Source: CAD feature listing. Evaluate the final solid. Frame: model axes, mm. A direction names the side the tool comes from. Give positions to 0.01 mm unless a question says otherwise; leave off trailing zeros. Order: outer loops, then holes, each group sorted by start corner. A loop starts at its lowest first (then second) coordinate and runs counter-clockwise, first axis right, second up. Notation, with made-up numbers: M 45,38 L 73,38 A20 cw 73,74 Z; hole C -7.5,-11 d5. An arc over 180 degrees is marked long. Return JSON: item names as keys, results as strings.
from build123d import *

# Parameters (mm, degrees)
SKETCH1_W           = 440
SKETCH1_H           = 170
BOSS_EXTRUDE1_DEPTH = 25
SKETCH2_R           = 9.5
CUT_EXTRUDE1_DEPTH  = 15
SKETCH4_R           = 6
CUT_EXTRUDE3_DEPTH  = 237.326045962
SKETCH3_R           = 9.5
CUT_EXTRUDE2_DEPTH  = 15
SKETCH5_R           = 6
CUT_EXTRUDE4_DEPTH  = 237.326045962


with BuildPart() as part:
    # Sketch1 → Boss-Extrude1 (new body)
    with BuildSketch(Plane.XY):
        Rectangle(SKETCH1_W, SKETCH1_H)
    extrude(amount=BOSS_EXTRUDE1_DEPTH)

    # Sketch2 → Cut-Extrude1 (cut)
    with BuildSketch(Plane.XY.offset(25)):
        with Locations((170, 65)):
            Circle(SKETCH2_R)
        with Locations((45, 65)):
            Circle(SKETCH2_R)
        with Locations((-80, 65)):
            Circle(SKETCH2_R)
        with Locations((-205, 65)):
            Circle(SKETCH2_R)
        with Locations((45, -60)):
            Circle(SKETCH2_R)
        with Locations((-80, -60)):
            Circle(SKETCH2_R)
        with Locations((-205, -60)):
            Circle(SKETCH2_R)
        with Locations((170, -60)):
            Circle(SKETCH2_R)
    extrude(amount=-CUT_EXTRUDE1_DEPTH, mode=Mode.SUBTRACT)

    # Sketch4 → Cut-Extrude3 (cut, through all)
    with BuildSketch(Plane.XY.offset(10)):
        with Locations((170, 65)):
            Circle(SKETCH4_R)
        with Locations((45, 65)):
            Circle(SKETCH4_R)
        with Locations((-80, 65)):
            Circle(SKETCH4_R)
        with Locations((-205, 65)):
            Circle(SKETCH4_R)
        with Locations((45, -60)):
            Circle(SKETCH4_R)
        with Locations((-80, -60)):
            Circle(SKETCH4_R)
        with Locations((-205, -60)):
            Circle(SKETCH4_R)
        with Locations((170, -60)):
            Circle(SKETCH4_R)
    extrude(amount=-CUT_EXTRUDE3_DEPTH, mode=Mode.SUBTRACT)

    # Sketch3 → Cut-Extrude2 (cut)
    with BuildSketch(Plane(origin=(0, 0, 0), x_dir=(-1, 0, 0), z_dir=(0, 0, -1))):
        with Locations((-107.5, -60)):
            Circle(SKETCH3_R)
        with Locations((17.5, -60)):
            Circle(SKETCH3_R)
        with Locations((142.5, -60)):
            Circle(SKETCH3_R)
        with Locations((17.5, 65)):
            Circle(SKETCH3_R)
        with Locations((142.5, 65)):
            Circle(SKETCH3_R)
        with Locations((-107.5, 65)):
            Circle(SKETCH3_R)
    extrude(amount=-CUT_EXTRUDE2_DEPTH, mode=Mode.SUBTRACT)

    # Sketch5 → Cut-Extrude4 (cut, through all)
    with BuildSketch(Plane(origin=(0, 0, 15), x_dir=(-1, 0, 0), z_dir=(0, 0, -1))):
        with Locations((-107.5, -60)):
            Circle(SKETCH5_R)
        with Locations((17.5, -60)):
            Circle(SKETCH5_R)
        with Locations((142.5, -60)):
            Circle(SKETCH5_R)
        with Locations((17.5, 65)):
            Circle(SKETCH5_R)
        with Locations((142.5, 65)):
            Circle(SKETCH5_R)
        with Locations((-107.5, 65)):
            Circle(SKETCH5_R)
    extrude(amount=-CUT_EXTRUDE4_DEPTH, mode=Mode.SUBTRACT)


solid = part.part
1. Section query A-A (x = -17.5). Return loops of the section in (y, z).
Evaluation:
{"outline": "M -85,0 L -69.5,0 L -69.5,15 L -66,15 L -66,25 L -85,25 Z; M -54,15 L -50.5,15 L -50.5,0 L 55.5,0 L 55.5,15 L 59,15 L 59,25 L -54,25 Z; M 71,15 L 74.5,15 L 74.5,0 L 85,0 L 85,25 L 71,25 Z"}
2. Ray query, probe 1 along Y at (x, z) = (170, 14); probe 2 along Y at (x, z) = (45, 2). Return the intervals inside material, ascending.
Evaluation:
{"probe 1": "y = -85 to -69.5, -50.5 to 55.5, 74.5 to 85", "probe 2": "y = -85 to -66, -54 to 59, 71 to 85"}
3. First-contact query: pin 1 (15 mm diameter, centred on x = -142.5, y = 65, fed in from -Z); pin 2 (15.5 mm diameter, centred on x = -80, y = -60, fed in from +Z). Flat tips, straight axial feed; report the tip coordinate or a pass-through.
Evaluation:
{"pin 1": "stops at z = 15", "pin 2": "stops at z = 10"}
4. Set-up query: faces 3 (the face through (175.11, 73.01, 17.6)), 4 (the face through (-137.74, -63.65, 19.93)), 5 (the face through (-17.4, 58.8, 15)). Return all of +Z, -Z, +X, -X, +Y, -Y with unobstructed straight access to the full face (end or side cutting, diameter ignored); none if empty.
Evaluation:
{"face 3": "+Z", "face 4": "+Z, -Z", "face 5": "-Z"}
5. Draft query along X for faces 1 (the face through (-3, 85, 12)), 2 (the face through (-138.08, 69.06, 19.93)). Return one class per face: pulls with the +X half, pulls with the -X half, needs draft (parallel to the pull), parting line crosses it, or undercut.
Evaluation:
{"face 1": "needs draft", "face 2": "undercut"}
6. Section query B-B (z = 5.25). State how many separate pieces and enclosed holes the cut face has, then the cut area to 3 significant figures.
Evaluation:
{"separate pieces": "1", "enclosed holes": "14", "area": "72,200 mm^2"}
